Geometry: final body of the model. Coordinates: model frame, mm. Coordinates: 2 decimals unless noted, no trailing zeros. Loops run counter-clockwise (first coordinate to the right, second up) from the corner with the lowest first, then second, coordinate; pieces in that order, holes last. Notation, with made-up numbers: (-22, 25.5) - (-5, 25.5) arc R11 cw to (-5, 38.5) - close; hole circle Ø4 at (66, -13). An arc over 180 degrees is marked (long way). Put each result on its own line as item: value. Start each with the question number.
1) Material intervals for line 1 along Z through (x, y) = (42, 0.3); line 2 along Z through (x, y) = (40.5, 0.55); line 3 along X through (y, z) = (0.2, -14), sorted ascending. Write a range as from..to.
2) Contact query for a flat-ended pin moving along its axis: pin 1 Ø0.5 at (y, z) = (0.5, -54) entering from -X. Output: stop coordinate, or through.
3) Draft query along X for faces 1 (the flat face through (51, 0, 2)), 2 (the cylindrical face through (46.326, 0.493, 77.257)), 3 (the cylindrical face through (66.874, 0.493, -63.475)), 4 (the cylindrical face through (37.285, 0.493, -78.404)). Return one class per face: +X half, -X half, draft (parallel to the pull), parting line (faces both ways), or undercut.
4) Section A-A on y = 0.7. Output: boundary loops of the cut face in (x, z).
5) Section C-C on z = -26. Output: boundary loops of the cut face in (x, y).
Autodesk Inventor part; units mm, degrees
ref_plane "YZ Plane" through (0, 0, 0) normal (1, 0, 0) x (0, 1, 0)
ref_plane "XZ Plane" through (0, 0, 0) normal (0, 1, 0) x (-1, 0, 0)
ref_plane "XY Plane" through (0, 0, 0) normal (0, 0, 1) x (1, 0, 0)
sketch "Esboço1" plane through (0, 0, 0) normal (0, 1, 0) x (-1, 0, 0)
  line L0 (-30.1128, 0) -> (-45.5357, 0)
  line L1 (-34.1868, -120) -> (-40.1868, -120)
  arc A0 (-76.9634, 0) -> (-40.1868, -120) centre (147.3829, 3.1204) ccw
  line L2 (-34.1868, -67.7964) -> (-45.5357, -67.7964)
  line L3 (-45.5357, -67.7964) -> (-45.5357, -41.1109)
  line L4 (-45.5357, -41.1109) -> (-34.1868, -41.1109)
  line L5 (-34.1868, 0) -> (-34.1868, -41.1109)
  line L6 (-34.1868, -67.7964) -> (-34.1868, -120)
  circle A1 centre (-38.629, -76.2964) radius 2.5
  circle A2 centre (-38.629, -76.2964) radius 2.5
  circle A3 centre (-48.643, -76.2964) radius 2.5086
  line L7 (-34.1868, 120) -> (-40.1868, 120)
  arc A4 (-40.1868, 120) -> (-76.9634, 0) centre (147.3829, -3.1204) ccw
  line L8 (-34.1868, 67.7964) -> (-45.5357, 67.7964)
  line L9 (-45.5357, 67.7964) -> (-45.5357, 41.1109)
  line L10 (-45.5357, 41.1109) -> (-34.1868, 41.1109)
  line L11 (-34.1868, 0) -> (-34.1868, 41.1109)
  line L12 (-34.1868, 67.7964) -> (-34.1868, 120)
  circle A5 centre (-38.629, 76.2964) radius 2.5
  circle A6 centre (-48.643, 76.2964) radius 2.5086
  point P0 (0, 0)
  point P1 (0, 0)
  dimension "d0" = 120
  dimension "d1" = 6
extrude "Extrusão1" add sketch "Esboço1" along normal blind 1
sketch "Esboço2" plane through (0, 0, 0) normal (0, 1, 0) x (-1, 0, 0)
  point P0 (0, 0)
sketch "Esboço3" plane through (0, 0, 0) normal (0, -1, 0) x (1, 0, 0)
  line L0 (45.5357, 41.1109) -> (45.5357, 67.7964)
  line L1 (45.5357, 41.1109) -> (45.5357, 52.7605)
  point P0 (0, 0)
properties part number "sensores1"
Answer block:
1. line 1: z = -117.19..-67.8, -41.11..41.11, 67.8..117.19
1. line 2: z = -119.52..-77.95, -74.64..-67.8, -41.11..41.11, 67.8..74.64, 77.95..119.52
1. line 3: x = 34.19..76.33
2. pin 1: stops at x = 45.54
3. face 1: draft
3. face 2: undercut
3. face 3: +X half
3. face 4: undercut
4. outline: (34.19, -120) - (40.19, -120) arc R224.37 ccw to (76.96, 0) arc R224.37 ccw to (40.19, 120) - (34.19, 120) - (34.19, 67.8) - (45.54, 67.8) - (45.54, 41.11) - (34.19, 41.11) - (34.19, -41.11) - (45.54, -41.11) - (45.54, -67.8) - (34.19, -67.8) - close; hole circle Ø5 at (38.63, -76.3); hole circle Ø5 at (38.63, 76.3); hole circle Ø5.02 at (48.64, -76.3); hole circle Ø5.02 at (48.64, 76.3)
5. outline: (34.19, 0) - (75.09, 0) - (75.09, 1) - (34.19, 1) - close
